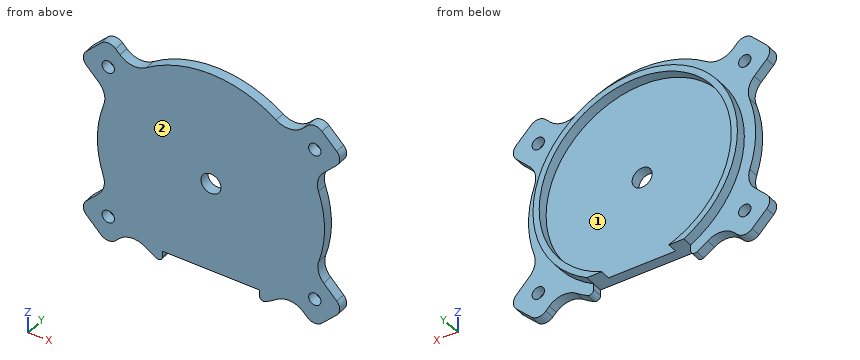
from build123d import *

# Parameters (mm, degrees)
SKETCH_1_R                  = 55
EXTRUDE_1_DEPTH             = 5
SKETCH_5_W                  = 47
SKETCH_5_H                  = 12.24289715
CUT_EXTRUDE_2_DEPTH         = 30
FILLET_4_R                  = 2
FILLET_5_R                  = 2
EXTRUDE_3_REACH             = 79.84
EXTRUDE_3_DIRECTION_2_REACH = 79.84
FILLET_7_R                  = 10
FILLET_8_R                  = 5
SKETCH_10_R                 = 3
CUT_EXTRUDE_5_DEPTH         = 5
SKETCH_15_R                 = 4.85
CUT_EXTRUDE_6_DEPTH         = 10
EXTRUDE_4_DEPTH             = 5


with BuildPart() as part:
    # 草图1 → 凸台-拉伸1 (new body)
    with BuildSketch(Plane(origin=(0, 0, 0), x_dir=(1, 0, 0), z_dir=(0, 1, 0))):
        with Locations(Location((0, 0, 0), (0, 0, 270))):
            Circle(SKETCH_1_R)
    extrude(amount=EXTRUDE_1_DEPTH)

    # 草图5 → 切除-拉伸2 (cut)
    with BuildSketch(Plane(origin=(0, 5, 0), x_dir=(1, 0, 0), z_dir=(0, 1, 0))):
        with Locations((0, 49.687490397)):
            Rectangle(SKETCH_5_W, SKETCH_5_H)
    extrude(amount=-CUT_EXTRUDE_2_DEPTH, mode=Mode.SUBTRACT)

    # 圆角4
    fillet_4_edges = [part.edges().sort_by_distance(p)[0] for p in [
        (-23.5, 2.5, -49.726753363),
    ]]
    fillet(fillet_4_edges, radius=FILLET_4_R)

    # 圆角5
    fillet_5_edges = [part.edges().sort_by_distance(p)[0] for p in [
        (23.5, 2.5, -49.726753363),
    ]]
    fillet(fillet_5_edges, radius=FILLET_5_R)

    # 凸台-拉伸3: up to this face of the body (flat: up to its plane)
    extrude_3_end = Plane(part.part.faces().sort_by_distance((0, 0, 2.477505486))[0])
    # 草图14 → 凸台-拉伸3 (add, up to the picked face)
    with BuildSketch(Plane(origin=(0, 3, 0), x_dir=(1, 0, 0), z_dir=(0, 1, 0)), mode=Mode.PRIVATE) as extrude_3_sk1:
        with BuildLine():
            Line((-49.898576095, 23.132922507), (-63.862525635, 37.044772973))
            Line((-63.862525635, 37.044772973), (-49.746845912, 51.213315099))
            Line((-49.746845912, 51.213315099), (-38.128637352, 39.638453724))
            ThreePointArc((-38.128637352, 39.638453724), (-44.78063998, 31.932652301), (-49.898576095, 23.132922507))
        make_face()
    extrude_3_tool1 = split(extrude(extrude_3_sk1.sketch, amount=-EXTRUDE_3_REACH, mode=Mode.PRIVATE), bisect_by=extrude_3_end, keep=Keep.BOTH, mode=Mode.PRIVATE)
    # 草图14 → 凸台-拉伸3 (add, up to the picked face)
    with BuildSketch(Plane(origin=(0, 3, 0), x_dir=(1, 0, 0), z_dir=(0, 1, 0)), mode=Mode.PRIVATE) as extrude_3_sk2:
        with BuildLine():
            Line((49.811900188, -23.3189751), (64.421720913, -37.928795825))
            Line((64.421720913, -37.928795825), (50.279585289, -52.070931449))
            Line((50.279585289, -52.070931449), (37.984884655, -39.776230814))
            ThreePointArc((37.984884655, -39.776230814), (44.662950793, -32.097053236), (49.811900188, -23.3189751))
        make_face()
    extrude_3_tool2 = split(extrude(extrude_3_sk2.sketch, amount=-EXTRUDE_3_REACH, mode=Mode.PRIVATE), bisect_by=extrude_3_end, keep=Keep.BOTH, mode=Mode.PRIVATE)
    # 草图14 → 凸台-拉伸3 (add, up to the picked face)
    with BuildSketch(Plane(origin=(0, 3, 0), x_dir=(1, 0, 0), z_dir=(0, 1, 0)), mode=Mode.PRIVATE) as extrude_3_sk3:
        with BuildLine():
            Line((-49.632393674, -23.698639164), (-63.862550335, -37.928795825))
            Line((-63.862550335, -37.928795825), (-49.720414711, -52.070931449))
            Line((-49.720414711, -52.070931449), (-37.697852746, -40.048369484))
            ThreePointArc((-37.697852746, -40.048369484), (-44.423770724, -32.427281642), (-49.632393674, -23.698639164))
        make_face()
    extrude_3_tool3 = split(extrude(extrude_3_sk3.sketch, amount=-EXTRUDE_3_REACH, mode=Mode.PRIVATE), bisect_by=extrude_3_end, keep=Keep.BOTH, mode=Mode.PRIVATE)
    # 草图14 → 凸台-拉伸3 (add, up to the picked face)
    with BuildSketch(Plane(origin=(0, 3, 0), x_dir=(1, 0, 0), z_dir=(0, 1, 0)), mode=Mode.PRIVATE) as extrude_3_sk4:
        with BuildLine():
            Line((38.475737251, 39.301623923), (50.118901666, 51.212426922))
            Line((50.118901666, 51.212426922), (64.420808036, 37.231887798))
            Line((64.420808036, 37.231887798), (50.134465219, 22.6171483))
            ThreePointArc((50.134465219, 22.6171483), (45.083643676, 31.50341367), (38.475737251, 39.301623923))
        make_face()
    extrude_3_tool4 = split(extrude(extrude_3_sk4.sketch, amount=-EXTRUDE_3_REACH, mode=Mode.PRIVATE), bisect_by=extrude_3_end, keep=Keep.BOTH, mode=Mode.PRIVATE)
    add(extrude_3_tool1.solids().sort_by(Axis((-50.837096, 3, -37.73966), (0, -1, 0)))[0])
    add(extrude_3_tool2.solids().sort_by(Axis((51.039653, 3, 38.272151), (0, -1, 0)))[0])
    add(extrude_3_tool3.solids().sort_by(Axis((-50.639154, 3, 38.439997), (0, -1, 0)))[0])
    add(extrude_3_tool4.solids().sort_by(Axis((51.238479, 3, -37.552164), (0, -1, 0)))[0])

    # 凸台-拉伸3 direction 2: up to this face of the body (flat: up to its plane)
    extrude_3_direction_2_end = Plane(part.part.faces().sort_by_distance((0, 5, 2.477505486))[0])
    # 草图14 → 凸台-拉伸3 direction 2 (add, up to the picked face)
    with BuildSketch(Plane(origin=(0, 3, 0), x_dir=(1, 0, 0), z_dir=(0, 1, 0)), mode=Mode.PRIVATE) as extrude_3_direction_2_sk1:
        with BuildLine():
            Line((-49.898576095, 23.132922507), (-63.862525635, 37.044772973))
            Line((-63.862525635, 37.044772973), (-49.746845912, 51.213315099))
            Line((-49.746845912, 51.213315099), (-38.128637352, 39.638453724))
            ThreePointArc((-38.128637352, 39.638453724), (-44.78063998, 31.932652301), (-49.898576095, 23.132922507))
        make_face()
    extrude_3_direction_2_tool1 = split(extrude(extrude_3_direction_2_sk1.sketch, amount=EXTRUDE_3_DIRECTION_2_REACH, mode=Mode.PRIVATE), bisect_by=extrude_3_direction_2_end, keep=Keep.BOTH, mode=Mode.PRIVATE)
    # 草图14 → 凸台-拉伸3 direction 2 (add, up to the picked face)
    with BuildSketch(Plane(origin=(0, 3, 0), x_dir=(1, 0, 0), z_dir=(0, 1, 0)), mode=Mode.PRIVATE) as extrude_3_direction_2_sk2:
        with BuildLine():
            Line((49.811900188, -23.3189751), (64.421720913, -37.928795825))
            Line((64.421720913, -37.928795825), (50.279585289, -52.070931449))
            Line((50.279585289, -52.070931449), (37.984884655, -39.776230814))
            ThreePointArc((37.984884655, -39.776230814), (44.662950793, -32.097053236), (49.811900188, -23.3189751))
        make_face()
    extrude_3_direction_2_tool2 = split(extrude(extrude_3_direction_2_sk2.sketch, amount=EXTRUDE_3_DIRECTION_2_REACH, mode=Mode.PRIVATE), bisect_by=extrude_3_direction_2_end, keep=Keep.BOTH, mode=Mode.PRIVATE)
    # 草图14 → 凸台-拉伸3 direction 2 (add, up to the picked face)
    with BuildSketch(Plane(origin=(0, 3, 0), x_dir=(1, 0, 0), z_dir=(0, 1, 0)), mode=Mode.PRIVATE) as extrude_3_direction_2_sk3:
        with BuildLine():
            Line((-49.632393674, -23.698639164), (-63.862550335, -37.928795825))
            Line((-63.862550335, -37.928795825), (-49.720414711, -52.070931449))
            Line((-49.720414711, -52.070931449), (-37.697852746, -40.048369484))
            ThreePointArc((-37.697852746, -40.048369484), (-44.423770724, -32.427281642), (-49.632393674, -23.698639164))
        make_face()
    extrude_3_direction_2_tool3 = split(extrude(extrude_3_direction_2_sk3.sketch, amount=EXTRUDE_3_DIRECTION_2_REACH, mode=Mode.PRIVATE), bisect_by=extrude_3_direction_2_end, keep=Keep.BOTH, mode=Mode.PRIVATE)
    # 草图14 → 凸台-拉伸3 direction 2 (add, up to the picked face)
    with BuildSketch(Plane(origin=(0, 3, 0), x_dir=(1, 0, 0), z_dir=(0, 1, 0)), mode=Mode.PRIVATE) as extrude_3_direction_2_sk4:
        with BuildLine():
            Line((38.475737251, 39.301623923), (50.118901666, 51.212426922))
            Line((50.118901666, 51.212426922), (64.420808036, 37.231887798))
            Line((64.420808036, 37.231887798), (50.134465219, 22.6171483))
            ThreePointArc((50.134465219, 22.6171483), (45.083643676, 31.50341367), (38.475737251, 39.301623923))
        make_face()
    extrude_3_direction_2_tool4 = split(extrude(extrude_3_direction_2_sk4.sketch, amount=EXTRUDE_3_DIRECTION_2_REACH, mode=Mode.PRIVATE), bisect_by=extrude_3_direction_2_end, keep=Keep.BOTH, mode=Mode.PRIVATE)
    add(extrude_3_direction_2_tool1.solids().sort_by(Axis((-50.837096, 3, -37.73966), (0, 1, 0)))[0])
    add(extrude_3_direction_2_tool2.solids().sort_by(Axis((51.039653, 3, 38.272151), (0, 1, 0)))[0])
    add(extrude_3_direction_2_tool3.solids().sort_by(Axis((-50.639154, 3, 38.439997), (0, 1, 0)))[0])
    add(extrude_3_direction_2_tool4.solids().sort_by(Axis((51.238479, 3, -37.552164), (0, 1, 0)))[0])

    # 圆角7
    fillet_7_edges = [part.edges().sort_by_distance(p)[0] for p in [
        (-38.128637352, 2.5, -39.638453724),
        (-49.898576095, 2.5, -23.132922507),
        (-49.632393674, 2.5, 23.698639164),
        (-37.697852746, 2.5, 40.048369484),
        (50.134465219, 2.5, -22.6171483),
        (38.475737251, 2.5, -39.301623923),
        (37.984884655, 2.5, 39.776230814),
        (49.811900188, 2.5, 23.3189751),
    ]]
    fillet(fillet_7_edges, radius=FILLET_7_R)

    # 圆角8
    fillet_8_edges = [part.edges().sort_by_distance(p)[0] for p in [
        (-63.862525635, 2.5, -37.044772973),
        (-49.746845912, 2.5, -51.213315099),
        (-49.720414711, 2.5, 52.070931449),
        (-63.862550335, 2.5, 37.928795825),
        (50.118901666, 2.5, -51.212426922),
        (64.420808036, 2.5, -37.231887798),
        (50.279585289, 2.5, 52.070931449),
        (64.421720913, 2.5, 37.928795825),
    ]]
    fillet(fillet_8_edges, radius=FILLET_8_R)

    # 草图10 → 切除-拉伸5 (cut, symmetric)
    with BuildSketch(Plane(origin=(0, 3, 0), x_dir=(1, 0, 0), z_dir=(0, 1, 0))):
        with Locations(Location((-49.720414711, 37.071204175, 0), (0, 0, 270))):
            Circle(SKETCH_10_R)
        with Locations(Location((50.279585289, 37.071204175, 0), (0, 0, 270))):
            Circle(SKETCH_10_R)
        with Locations(Location((-49.720414711, -37.928795825, 0), (0, 0, 270))):
            Circle(SKETCH_10_R)
        with Locations(Location((50.279585289, -37.928795825, 0), (0, 0, 270))):
            Circle(SKETCH_10_R)
    extrude(amount=CUT_EXTRUDE_5_DEPTH, both=True, mode=Mode.SUBTRACT)

    # 草图15 → 切除-拉伸6 (cut)
    with BuildSketch(Plane(origin=(0, 5, 0), x_dir=(1, 0, 0), z_dir=(0, 1, 0))):
        with Locations(Location((0, 0, 0), (0, 0, 270))):
            Circle(SKETCH_15_R)
    extrude(amount=-CUT_EXTRUDE_6_DEPTH, mode=Mode.SUBTRACT)

    # 草图17 → 凸台-拉伸4 (add)
    with BuildSketch(Plane(origin=(0, 5, 0), x_dir=(1, 0, 0), z_dir=(0, 1, 0))):
        with BuildLine():
            Line((-23.5, 43.566041822), (-16.255768207, 43.566041822))
            ThreePointArc((-16.255768207, 43.566041822), (0, -46.5), (16.255768207, 43.566041822))
            Line((16.255768207, 43.566041822), (23.5, 43.566041822))
            ThreePointArc((23.5, 43.566041822), (0, -49.5), (-23.5, 43.566041822))
        make_face()
    extrude(amount=EXTRUDE_4_DEPTH)


solid = part.part
Read the model definition and answer for the solid it produces. Units are mm, in the model's axes. Face numbers are marked on the shaded views. Give positions to 0.01 mm unless a question says otherwise; leave off trailing zeros. Write each loop counter-clockwise with the first axis right and the second up, starting at its lowest first coordinate (ties: lowest second). Pieces come first, ordered by that corner, then holes. Notation, with made-up numbers: (9.25, 22) - (13.25, 22) arc R23 cw to (13.25, 36) - close; hole circle Ø1 at (39.5, 20.25). An arc over 180 degrees is marked (long way). Answer in a Markdown table with one row per item. Add a question column.
Item 1: Find the intervals of material crossed by L1, parallel to X at y = 4, z = -35; L2, parallel to X at y = 4.75, z = -39; L3, parallel to X at y = 2.7, z = 0, in increasing order.
Item 2: Determine the mould class of the marked faces 1 and 2 for opening direction Z: pulls with the +Z half, pulls with the -Z half, needs draft (parallel to the pull), parting line crosses it, or undercut.
Item 3: Section A-A, the plane x = 0 is taken. Write down the section's boundary in (y, z), and give its area (3 significant figures).
Item 4: Flat-ended cylindrical pins translate along their axes: P1, Ø7, axis at x = -49.72, z = 37.93, coming from the -Y side; P2, Ø7, axis at x = 50.28, z = -37.07, coming from the +Y side; P3, Ø0.9, axis at y = 2.5, z = -45.5, coming from the +X side; P4, Ø6, axis at y = 5.5, z = -29.5, coming from the -X side. Find the tip coordinate at first contact, or state that the pin passes through.
Item 5: Section D-D, the plane x = 18.5 is taken. Write down the section's boundary in (y, z).
Item 6: Section B-B, the plane z = 0 is taken. Write down the section's boundary in (x, y), and give its area (4 significant figures).
Item 7: Section C-C, the plane y = 2.75 is taken. Count the separate pieces of the cut face and the enclosed holes in it, and give its area (3 significant figures).
Recorded:
| question | item | result |
|---|---|---|
| 1 | L1 | x = -61.35 to -51.89, -47.55 to 48.11, 52.45 to 61.86 |
| 1 | L2 | x = -61.4 to -52.02, -47.42 to 47.98, 52.58 to 62 |
| 1 | L3 | x = -55 to -4.85, 4.85 to 55 |
| 2 | face 1 | undercut |
| 2 | face 2 | needs draft |
| 3 | outline | (0, -43.57) - (5, -43.57) - (5, -4.85) - (0, -4.85) - close; (0, 4.85) - (5, 4.85) - (5, 46.5) - (10, 46.5) - (10, 49.5) - (5, 49.5) - (5, 55) - (0, 55) - close |
| 3 | area | 459 mm2 |
| 4 | P1 | stops at y = 0 |
| 4 | P2 | stops at y = 5 |
| 4 | P3 | stops at x = 56.42 |
| 4 | P4 | stops at x = -59.26 |
| 5 | outline | (0, -43.57) - (10, -43.57) - (10, -42.66) - (5, -42.66) - (5, 42.66) - (10, 42.66) - (10, 45.91) - (5, 45.91) - (5, 51.8) - (0, 51.8) - close |
| 6 | outline | (-55, 0) - (-4.85, 0) - (-4.85, 5) - (-46.5, 5) - (-46.5, 10) - (-49.5, 10) - (-49.5, 5) - (-55, 5) - close; (4.85, 0) - (55, 0) - (55, 5) - (49.5, 5) - (49.5, 10) - (46.5, 10) - (46.5, 5) - (4.85, 5) - close |
| 6 | area | 531.5 mm2 |
| 7 | separate pieces | 1 |
| 7 | enclosed holes | 5 |
| 7 | area | 10,300 mm2 |
